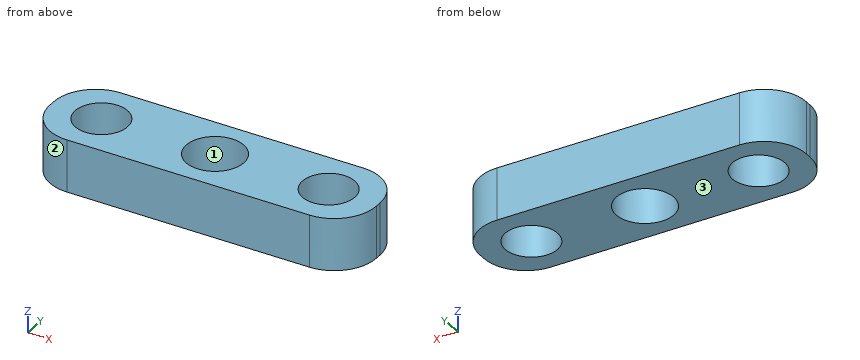
```python
from build123d import *

# Parameters (mm, degrees)
SKETCH1_W           = 15.555334961
SKETCH1_H           = 8.618657178
SKETCH1_R           = 2.5
BOSS_EXTRUDE1_DEPTH = 5
SKETCH2_R           = 2.75
CUT_EXTRUDE1_DEPTH  = 22.76046651
FILLET1_R           = 4


with BuildPart() as part:
    # Sketch1 → Boss-Extrude1 (new body)
    # profile 1 of 2: a face of its own
    with BuildSketch(Plane.XY):
        with Locations((-7.777667481, 10.0625)):
            Rectangle(SKETCH1_W, SKETCH1_H)
        with Locations((-10.828492502, 10.0625)):
            Circle(SKETCH1_R, mode=Mode.SUBTRACT)
    # profile 2 of 2: a face of its own
    with BuildSketch(Plane.XY):
        with Locations((7.777667481, 10.0625)):
            Rectangle(SKETCH1_W, SKETCH1_H)
        with Locations((10.828492502, 10.0625)):
            Circle(SKETCH1_R, mode=Mode.SUBTRACT)
    extrude(amount=BOSS_EXTRUDE1_DEPTH)

    # Sketch2 → Cut-Extrude1 (cut, through all)
    with BuildSketch(Plane.XY.offset(5)):
        with Locations((0, 10.0625)):
            Circle(SKETCH2_R)
    extrude(amount=-CUT_EXTRUDE1_DEPTH, mode=Mode.SUBTRACT)

    # Fillet1
    fillet1_edges = [part.edges().sort_by_distance(p)[0] for p in [
        (15.555334961, 14.371828589, 2.5),
        (15.555334961, 5.753171411, 2.5),
        (-15.555334961, 5.753171411, 2.5),
        (-15.555334961, 14.371828589, 2.5),
    ]]
    fillet(fillet1_edges, radius=FILLET1_R)


solid = part.part
```
Could you check a few things on this model? Use its own coordinates, in mm. Face numbers are marked on the shaded views. Round coordinates to 2 decimals unless told otherwise and drop trailing zeros. Loops run counter-clockwise (first coordinate to the right, second up) from the corner with the lowest first, then second, coordinate; pieces in that order, holes last. Notation, with made-up numbers: (76.5, 63) - (85.5, 63) arc R31 cw to (85.5, 102) - close; hole circle Ø5 at (-15, 45.25). An arc over 180 degrees is marked (long way). Answer as CSV lines item,"result".
1. I want a section at B-B on y = 8. List the corners of the cut face in (x, z) for me.
Filled in:
outline,"(-15.15, 0) - (-12.24, 0) - (-12.24, 5) - (-15.15, 5) - close; (-9.42, 0) - (-1.82, 0) - (-1.82, 5) - (-9.42, 5) - close; (1.82, 0) - (9.42, 0) - (9.42, 5) - (1.82, 5) - close; (12.24, 0) - (15.15, 0) - (15.15, 5) - (12.24, 5) - close"
2. We'd pull the mould along X, two halves only. Please class the marked faces 1, 2 and 3: +X half, -X half, draft (parallel to the pull), parting line (faces both ways), or undercut.
Filled in:
face 1,"undercut"
face 2,"-X half"
face 3,"draft"
3. I want a section at D-D on x = -13. List the corners of the cut face in (y, z) for me, then the cut area to 3 significant figures.
Filled in:
outline,"(6.02, 0) - (8.82, 0) - (8.82, 5) - (6.02, 5) - close; (11.3, 0) - (14.1, 0) - (14.1, 5) - (11.3, 5) - close"
area,"28.0 mm^2"
4. Please list where these lines run through material, in increasing order: line 1 along X through (y, z) = (11, 2.6); line 2 along X through (y, z) = (8.5, 2.9); line 3 along Y through (x, z) = (11, 0.65). Write a range as [from, to].
Filled in:
line 1,"x = [-15.51, -13.15], [-8.51, -2.59], [2.59, 8.51], [13.15, 15.51]"
line 2,"x = [-15.35, -12.78], [-8.88, -2.26], [2.26, 8.88], [12.78, 15.35]"
line 3,"y = [5.75, 7.57], [12.56, 14.37]"
5. I want a section at C-C on z = 2.9. List the corners of the cut face in (x, y) for me.
Filled in:
outline,"(-15.56, 9.75) arc R4 ccw to (-11.56, 5.75) - (11.56, 5.75) arc R4 ccw to (15.56, 9.75) - (15.56, 10.37) arc R4 ccw to (11.56, 14.37) - (-11.56, 14.37) arc R4 ccw to (-15.56, 10.37) - close; hole circle Ø5 at (-10.83, 10.06); hole circle Ø5.5 at (0, 10.06); hole circle Ø5 at (10.83, 10.06)"
6. I want a section at A-A on x = 0. List the corners of the cut face in (y, z) for me, then the cut area to 3 significant figures.
Filled in:
outline,"(5.75, 0) - (7.31, 0) - (7.31, 5) - (5.75, 5) - close; (12.81, 0) - (14.37, 0) - (14.37, 5) - (12.81, 5) - close"
area,"15.6 mm^2"
7. For pin 1 Ø1.5 at (y, z) = (11.5, 2) entering from +X; pin 2 Ø3 at (y, z) = (7, 4) entering from +X, each with a flat end and sliding along its axis, tell me the tip position at first contact or that it passes through.
Filled in:
pin 1,"stops at x = 15.54"
pin 2,"stops at x = 15.35"
